Answer from the drawing. Dimensions are ordinates in mm from the lowest x, y and z of the part. A direction names the side the tool comes from. Coordinates: 2 decimals unless noted, no trailing zeros. Loops run counter-clockwise (first coordinate to the right, second up) from the corner with the lowest first, then second, coordinate; pieces in that order, holes last. Notation, with made-up numbers: M -25,71.5 L -6,71.5 A11 cw -6,90.5 Z; hole C 12,44 d10. An arc over 180 degrees is marked long. Put each result on its own line as item: value.
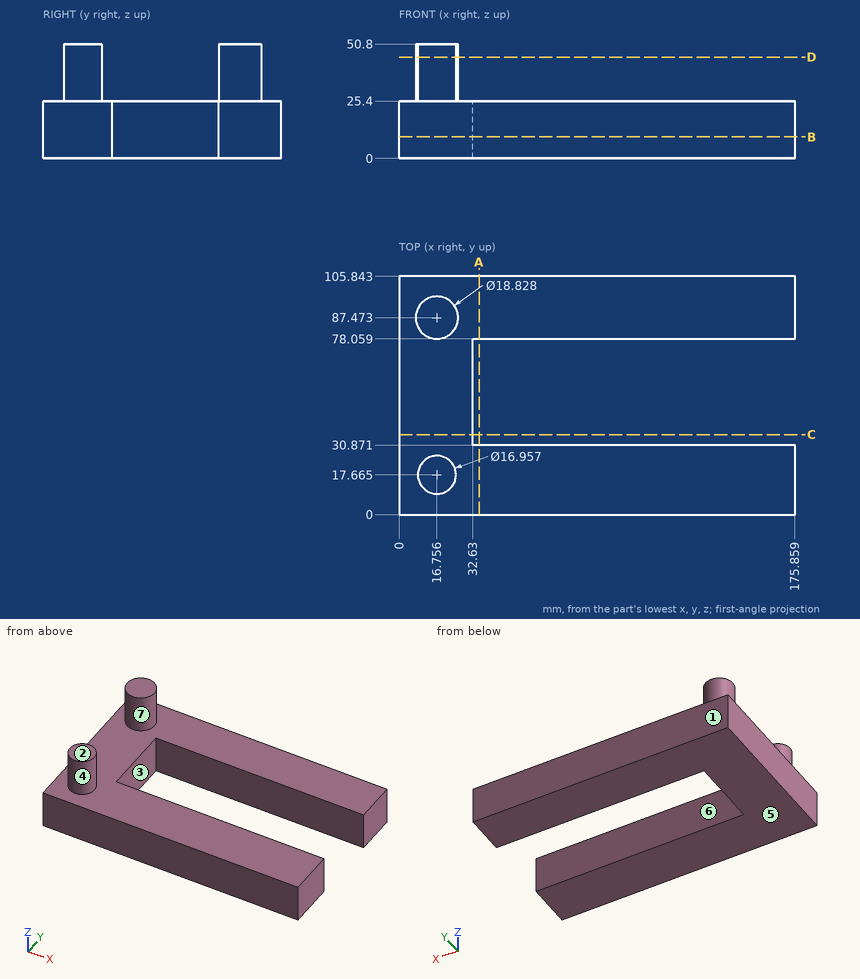
1) Find section C-C, the plane y = 35.5. Write down the section's boundary in (x, z), plus the area to 3 significant figures.
Answer list:
outline: M 0,0 L 32.63,0 L 32.63,25.4 L 0,25.4 Z
area: 829 mm^2
2) Find section D-D, the plane z = 45. Write down the section's boundary in (x, y) (1 decimal), plus the area to 3 significant figures.
Answer list:
outline: C 16.8,87.5 d18.8; C 16.8,17.7 d17
area: 504 mm^2
3) Straight lines are drawn through the part: line 1 (Y direction, x = 101, z = 6.5); line 2 (Z direction, x = 63, y = 91); line 3 (Y direction, x = 17, z = 30.5) (1 decimal). For each, find the intervals that lie inside material, in ascending order. Write a range as [from, to].
Answer list:
line 1: y = [0, 30.87], [78.06, 105.84]
line 2: z = [0, 25.4]
line 3: y = [9.2, 26.1], [78.1, 96.9]
4) Given pin 1 Ø6 at (x, y) = (18, 63.5) entering from +Z; pin 2 Ø8 at (y, z) = (44.5, 27) entering from +X; pin 3 Ø8 at (y, z) = (17, 37.5) entering from -X, each flat-ended and moving along its own axis, determine where each tip first touches the part or whether it passes through.
Answer list:
pin 1: stops at z = 25.4
pin 2: stops at x = 32.63
pin 3: stops at x = 8.28
5) Find section A-A, the plane x = 35.5. Write down the section's boundary in (y, z), plus the area to 3 significant figures.
Answer list:
outline: M 0,0 L 30.87,0 L 30.87,25.4 L 0,25.4 Z; M 78.06,0 L 105.84,0 L 105.84,25.4 L 78.06,25.4 Z
area: 1,490 mm^2
6) Determine the mould class of the marked faces 1, 2, 3 and 4 for opening direction Y: released by +Y, released by -Y, zero draft, split by the parting line, or undercut.
Answer list:
face 1: released by +Y
face 2: zero draft
face 3: undercut
face 4: undercut
7) Which of the six approach directions +Z, -Z, +X, -X, +Y, -Y give full straight-line access (tool end or side, diameter ignored) to the marked faces 5, 6 and 7?
Answer list:
face 5: -Z, +X, -X, +Y, -Y
face 6: +Z, -Z, +X
face 7: +Z
8) Find section B-B, the plane z = 9.5. Write down the section's boundary in (x, y).
Answer list:
outline: M 0,0 L 175.86,0 L 175.86,30.87 L 32.63,30.87 L 32.63,78.06 L 175.86,78.06 L 175.86,105.84 L 0,105.84 Z
